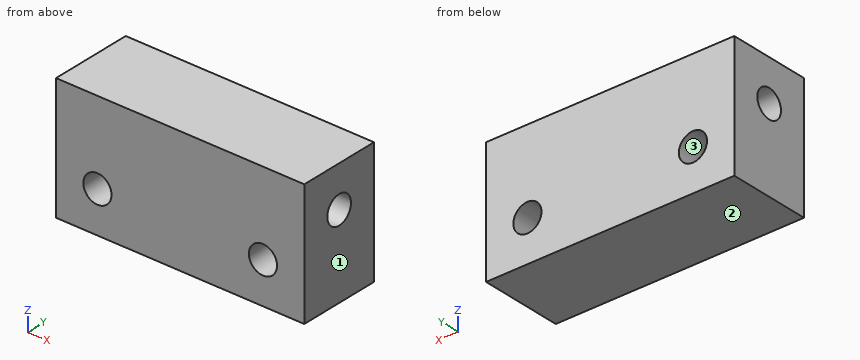
Autodesk Inventor part; units mm, degrees
ref_plane "YZ Plane" through (0, 0, 0) normal (1, 0, 0) x (0, 1, 0)
ref_plane "XZ Plane" through (0, 0, 0) normal (0, 1, 0) x (-1, 0, 0)
ref_plane "XY Plane" through (0, 0, 0) normal (0, 0, 1) x (1, 0, 0)
sketch "Sketch1" plane through (0, 0, 0) normal (1, 0, 0) x (0, 1, 0)
  line L0 (7.8254, 10.5896) -> (-4.8746, 10.5896)
  line L1 (-4.8746, 10.5896) -> (-4.8746, -8.4604)
  line L2 (-4.8746, -8.4604) -> (7.8254, -8.4604)
  line L3 (7.8254, -8.4604) -> (7.8254, 10.5896)
  point P0 (0, 0)
  dimension "d0" = 19.05
  dimension "d1" = 12.7
extrude "Extrusion1" add sketch "Sketch1" along normal blind 38.1
sketch "Sketch2" plane through (38.1, 0, 0) normal (1, 0, 0) x (0, 0, -1)
  line L0 (-10.5896, 7.8254) -> (-10.5896, -4.8746)
  line L1 (8.4604, 7.8254) -> (-10.5896, 7.8254)
  point P0 (0, 0)
  point P1 (-4.2396, 1.4754)
  dimension "d4" = 6.35
  dimension "d5" = 6.35
hole "Hole1" at (38.1, 1.4754, 4.2396) direction (-1, 0, 0) diameter 4.318 end through all
sketch "Sketch3" plane through (0, 7.8254, 10.5896) normal (0, 1, 0) x (1, 0, 0)
  line L0 (38.1, 19.05) -> (38.1, 0)
  line L1 (0, 19.05) -> (0, 0)
  line L2 (0, 19.05) -> (38.1, 19.05)
  point P0 (0, 10.5896)
  point P1 (6.35, 12.7)
  point P2 (31.75, 12.7)
  dimension "d13" = 6.35
  dimension "d14" = 6.35
  dimension "d15" = 6.35
  dimension "d16" = 0
hole "Hole2" at (6.35, 7.8254, -2.1104) at (31.75, 7.8254, -2.1104) direction (0, -1, 0) diameter 4.318 end through all
properties part number "MotorSpacerBlock2"
Geometry check sheet. Reference: the model listing, model coordinates, mm. Face numbers are marked on the shaded views. Give positions to 0.01 mm unless a question says otherwise; leave off trailing zeros. Loops run counter-clockwise (first coordinate to the right, second up) from the corner with the lowest first, then second, coordinate; pieces in that order, holes last. Notation, with made-up numbers: M 27.25,30.25 L 43.25,30.25 A22 ccw 43.25,46.25 Z; hole C 5,50.25 d4. An arc over 180 degrees is marked long. Write item = value, one per line. Start each with the question number.
1. Section check A-A, the plane x = 31. Enter the section's corners in (y, z).
2. Thickness scan on probe 1 along Z at (x, y) = (6.35, 0.25); probe 2 along X at (y, z) = (6, -2.25); probe 3 along Z at (x, y) = (6.35, 3). Record the ranges inside material, lowest first.
3. Go/stop test with a flat-tipped pin: P1, Ø5, axis at y = 1.48, z = 4.24, coming from the -X side. Record where the tip stops, or that it passes through.
4. Section check C-C, the plane z = -1. Enter the section's corners in (x, y), plus the area to 3 significant figures.
5. Section check D-D, the plane z = 3. Enter the section's corners in (x, y).
6. Section check B-B, the plane y = 2.5. Enter the section's corners in (x, z), plus the area to 3 significant figures.
7. Draft check along X on the marked faces 1, 2 and 3. Enter one of: +X half, -X half, draft (parallel to the pull), parting line (faces both ways), or undercut.
Values follow:
q1.outline = M -4.87,-8.46 L 7.83,-8.46 L 7.83,-4.13 L -4.87,-4.13 Z; M -4.87,-0.09 L 7.83,-0.09 L 7.83,10.59 L -4.87,10.59 Z; hole C 1.48,4.24 d4.32
q2.probe_1 = -8.46 to -4.27, 0.05 to 2.46, 6.02 to 10.59
q2.probe_2 = 0 to 4.2, 8.5 to 29.6, 33.9 to 38.1
q2.probe_3 = -8.46 to -4.27, 0.05 to 2.71, 5.77 to 10.59
q3.P1 = 0
q4.outline = M 0,-4.87 L 4.5,-4.87 L 4.5,7.83 L 0,7.83 Z; M 8.2,-4.87 L 29.9,-4.87 L 29.9,7.83 L 8.2,7.83 Z; M 33.6,-4.87 L 38.1,-4.87 L 38.1,7.83 L 33.6,7.83 Z
q4.area = 390 mm^2
q5.outline = M 0,-4.87 L 38.1,-4.87 L 38.1,-0.29 L 0,-0.29 Z; M 0,3.24 L 38.1,3.24 L 38.1,7.83 L 0,7.83 Z
q6.outline = M 0,-8.46 L 38.1,-8.46 L 38.1,2.34 L 0,2.34 Z; M 0,6.14 L 38.1,6.14 L 38.1,10.59 L 0,10.59 Z; hole C 6.35,-2.11 d4.32; hole C 31.75,-2.11 d4.32
q6.area = 552 mm^2
q7.face_1 = +X half
q7.face_2 = draft
q7.face_3 = undercut
